```python
from build123d import *

# Parameters (mm, degrees)
PAD_DEPTH   = 160
FILLET_R    = 6
FILLET001_R = 4.5
FILLET002_R = 6


with BuildPart() as part:
    # Sketch → Pad (new body)
    with BuildSketch(Plane.XY):
        Polygon((0, 0), (50, 0), (50, 8), (8, 8), (8, 20), (0, 20), align=None)
    extrude(amount=PAD_DEPTH)

    # Fillet
    fillet_edges = [part.edges().sort_by_distance(p)[0] for p in [
        (0, 0, 80),
    ]]
    fillet(fillet_edges, radius=FILLET_R)

    # Fillet001
    fillet001_edges = [part.edges().sort_by_distance(p)[0] for p in [
        (50, 8, 80),
        (8, 20, 80),
    ]]
    fillet(fillet001_edges, radius=FILLET001_R)

    # Fillet002
    fillet002_edges = [part.edges().sort_by_distance(p)[0] for p in [
        (8, 8, 80),
    ]]
    fillet(fillet002_edges, radius=FILLET002_R)


solid = part.part
```
The model under review builds one solid part; all positions refer to its coordinate system, in mm. A direction names the side the tool comes from. Round coordinates to 2 decimals unless told otherwise and drop trailing zeros. Loops run counter-clockwise (first coordinate to the right, second up) from the corner with the lowest first, then second, coordinate; pieces in that order, holes last.
1) Wall thickness on line 1 along Y through (x, z) = (17, 124); line 2 along X through (y, z) = (13.75, 121.5); line 3 along X through (y, z) = (5, 58): over which ranges is each line inside the solid? List them lowest first.
Values follow:
line 1: y = 0 to 8
line 2: x = 0 to 8.01
line 3: x = 0.08 to 49.74
2) Consider section C-C on y = 1.5. State the section outline as (x, z) points, then the cut area to 4 significant figures.
Values follow:
outline: (2.03, 0) - (50, 0) - (50, 160) - (2.03, 160) - close
area: 7,675 mm2
3) Consider section A-A on z = 72. State the section outline as (x, y) points, then the cut area to 3 significant figures.
Values follow:
outline: (0, 6) arc R6 ccw to (6, 0) - (50, 0) - (50, 3.5) arc R4.5 ccw to (45.5, 8) - (14, 8) arc R6 cw to (8, 14) - (8, 15.5) arc R4.5 ccw to (3.5, 20) - (0, 20) - close
area: 487 mm2
4) Tool access review of faces 1 (the face through (30, 8, 79)), 2 (the face through (2, 20, 79)): name each direction out of +Z, -Z, +X, -X, +Y, -Y from which nothing blocks a thin tool from reaching the whole face with its end or side.
Values follow:
face 1: +Z, -Z, +X, +Y
face 2: +Z, -Z, +X, -X, +Y
5) Consider section B-B on x = 18. State the section outline as (y, z) points, then the cut area to 3 significant figures.
Values follow:
outline: (0, 0) - (8, 0) - (8, 160) - (0, 160) - close
area: 1,280 mm2
6) Clearance check with flat-ended pins moving along their axes: P1, Ø4, axis at y = 15.5, z = 28.5, coming from the +X side; P2, Ø25, axis at x = 35, z = 116.5, coming from the +Y side; P3, Ø1.5, axis at y = 12, z = 118.5, coming from the +X side. State where each tip first meets the part, or that it passes through.
Values follow:
P1: stops at x = 8.02
P2: stops at y = 8
P3: stops at x = 8.67
